from build123d import *

# Parameters (mm, degrees)
SKETCH1_R           = 2.125
SKETCH1_W           = 19.725
SKETCH1_H           = 4
BOSS_EXTRUDE1_DEPTH = 4


with BuildPart() as part:
    # Sketch1 → Boss-Extrude1 (new body)
    with BuildSketch(Plane(origin=(0, 0, 0), x_dir=(1, 0, 0), z_dir=(0, 1, 0))):
        with BuildLine():
            Line((4, 0), (4, 20))
            Line((4, 20), (0, 20))
            Line((0, 20), (0, 40))
            Line((0, 40), (4, 40))
            Line((4, 40), (4, 60))
            Line((4, 60), (0, 60))
            Line((0, 60), (0, 80))
            Line((0, 80), (4, 80))
            Line((4, 80), (4, 100))
            Line((4, 100), (250, 100))
            Line((250, 100), (496, 100))
            Line((496, 100), (496, 80))
            Line((496, 80), (500, 80))
            Line((500, 80), (500, 60))
            Line((500, 60), (496, 60))
            Line((496, 60), (496, 40))
            Line((496, 40), (500, 40))
            Line((500, 40), (500, 20))
            Line((500, 20), (496, 20))
            Line((496, 20), (496, 0))
            Line((496, 0), (476, 0))
            Line((476, 0), (476, 1))
            ThreePointArc((476, 1), (459.890872965, 39.890872965), (421, 56))
            Line((421, 56), (79, 56))
            ThreePointArc((79, 56), (40.109127035, 39.890872965), (24, 1))
            Line((24, 1), (24, 0))
            Line((24, 0), (4, 0))
        make_face()
        with Locations((14, 15)):
            Circle(SKETCH1_R, mode=Mode.SUBTRACT)
        with Locations((14, 30)):
            Circle(SKETCH1_R, mode=Mode.SUBTRACT)
        with Locations((173.885, 90)):
            Circle(SKETCH1_R, mode=Mode.SUBTRACT)
        with Locations((326.115, 90)):
            Circle(SKETCH1_R, mode=Mode.SUBTRACT)
        with Locations((486, 30)):
            Circle(SKETCH1_R, mode=Mode.SUBTRACT)
        with Locations((486, 15)):
            Circle(SKETCH1_R, mode=Mode.SUBTRACT)
        with Locations((14, 60)):
            Circle(SKETCH1_R, mode=Mode.SUBTRACT)
        with Locations((14, 45)):
            Circle(SKETCH1_R, mode=Mode.SUBTRACT)
        with Locations((486, 45)):
            Circle(SKETCH1_R, mode=Mode.SUBTRACT)
        with Locations((486, 60)):
            Circle(SKETCH1_R, mode=Mode.SUBTRACT)
        with Locations((73.88, 66)):
            Circle(SKETCH1_R, mode=Mode.SUBTRACT)
        with Locations((426.12, 66)):
            Circle(SKETCH1_R, mode=Mode.SUBTRACT)
        with Locations((250, 66)):
            Circle(SKETCH1_R, mode=Mode.SUBTRACT)
        with Locations((63.3125, 78)):
            Rectangle(SKETCH1_W, SKETCH1_H, mode=Mode.SUBTRACT)
        with Locations((23.8625, 78)):
            Rectangle(SKETCH1_W, SKETCH1_H, mode=Mode.SUBTRACT)
        with Locations((102.7625, 78)):
            Rectangle(SKETCH1_W, SKETCH1_H, mode=Mode.SUBTRACT)
        with Locations((142.2125, 78)):
            Rectangle(SKETCH1_W, SKETCH1_H, mode=Mode.SUBTRACT)
        with Locations((181.6625, 78)):
            Rectangle(SKETCH1_W, SKETCH1_H, mode=Mode.SUBTRACT)
        with Locations((221.1125, 78)):
            Rectangle(SKETCH1_W, SKETCH1_H, mode=Mode.SUBTRACT)
        with Locations((278.8875, 78)):
            Rectangle(SKETCH1_W, SKETCH1_H, mode=Mode.SUBTRACT)
        with Locations((318.3375, 78)):
            Rectangle(SKETCH1_W, SKETCH1_H, mode=Mode.SUBTRACT)
        with Locations((357.7875, 78)):
            Rectangle(SKETCH1_W, SKETCH1_H, mode=Mode.SUBTRACT)
        with Locations((397.2375, 78)):
            Rectangle(SKETCH1_W, SKETCH1_H, mode=Mode.SUBTRACT)
        with Locations((436.6875, 78)):
            Rectangle(SKETCH1_W, SKETCH1_H, mode=Mode.SUBTRACT)
        with Locations((476.1375, 78)):
            Rectangle(SKETCH1_W, SKETCH1_H, mode=Mode.SUBTRACT)
    extrude(amount=BOSS_EXTRUDE1_DEPTH)


solid = part.part
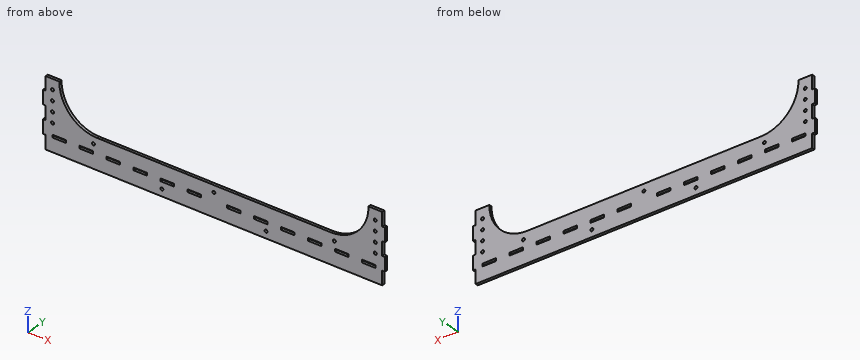
Could you check a few things on this model? Use its own coordinates, in mm. Coordinates: 2 decimals unless noted, no trailing zeros. Loops run counter-clockwise (first coordinate to the right, second up) from the corner with the lowest first, then second, coordinate; pieces in that order, holes last.
1. I need wall thicknesses on L1, parallel to X at y = 1.5, z = -66 (3 decimals); L2, parallel to Z at x = 392, y = 1.4; L3, parallel to X at y = 3, z = -30 (3 decimals). Which ranges of each line are inside material? Lowest first, please.
2. For P1, Ø2, axis at x = 2, y = 2.5, coming from the -Z side; P2, Ø2, axis at y = 2.5, z = -48.5, coming from the +X side, each with a flat end and sliding along its axis, tell me the tip position at first contact or that it passes through.
3. Imagine slicing it at B-B (x = 259). Please give me the cut outline in (y, z), and give its area (3 significant figures).
4. Imagine slicing it at A-A (y = 2.2). Give the number of separate pieces and of enclosed holes in the cut face, and give its area (3 significant figures).
Computed values:
1. L1: x = 0 to 71.755, 76.005 to 247.875, 252.125 to 423.995, 428.245 to 500
1. L2: z = -100 to -80, -76 to -56
1. L3: x = 0 to 11.875, 16.125 to 32.267, 467.733 to 483.875, 488.125 to 500
2. P1: stops at z = -80
2. P2: stops at x = 496
3. outline: (0, -100) - (4, -100) - (4, -56) - (0, -56) - close
3. area: 176 mm2
4. separate pieces: 1
4. enclosed holes: 25
4. area: 24,400 mm2
